Read the model definition and answer for the solid it produces. Units are mm, in the model's axes. A direction names the side the tool comes from. Give positions to 0.01 mm unless a question says otherwise; leave off trailing zeros. Loops run counter-clockwise (first coordinate to the right, second up) from the corner with the lowest first, then second, coordinate; pieces in that order, holes last. Notation, with made-up numbers: (48, 31.5) - (77, 31.5) arc R24 ccw to (77, 47.5) - close; hole circle Ø5 at (44.25, 70). An arc over 180 degrees is marked (long way). Put each result on its own line as item: value. Start each with the question number.
1. A cutting plane is placed at B-B, the plane x = 0. Determine the outline of the cut face in (y, z).
2. Given pin 1 Ø3 at (x, z) = (1.5, 74.5) entering from +Y; pin 2 Ø3 at (x, z) = (-1, 29.5) entering from -Y; pin 3 Ø6 at (y, z) = (-0.5, 71) entering from -X, each flat-ended and moving along its own axis, determine where each tip first touches the part or whether it passes through.
3. A cutting plane is placed at A-A, the plane y = -20. Determine the outline of the cut face in (x, z), plus the area to 3 significant figures.
4. For a pull along X with two mould halves and no side action, classify faces 1 (the flat face through (-3.901, 0, 49)), 2 (the flat face through (-8.2, -4, 49)), 3 (the flat face through (-4, 8.2, 49)), 4 (the flat face through (10, -10, 49)) as released by +X, released by -X, zero draft, split by the parting line, or undercut.
5. For faces 5 (the flat face through (0, -23.901, 49)), 6 (the flat face through (-9.11, -16.25, 49.3)), 7 (the flat face through (-7, -13.001, 51)), 8 (the flat face through (3.901, -20, 49)), determine the directions among +Z, -Z, +X, -X, +Y, -Y from which every point of the face is accessible in a straight line to the end or side of a thin tool.
6. Consider L1, parallel to Y at x = 0, z = 79.5; L2, parallel to Y at x = 6, z = 60; L3, parallel to Y at x = -5.25, z = 56. Determine where each line is inside the solid, lowest interval first. Write a range as from..to.
7. A cutting plane is placed at C-C, the plane z = 53. Count the separate pieces of the cut face and the enclosed holes in it, plus the area to 3 significant figures.
Autodesk Inventor part; units mm, degrees
ref_plane "Work Plane3" through (0, -20, 0) normal (0, 1, 0) x (-1, 0, 0)
ref_plane "YZ Plane" through (0, 0, 0) normal (1, 0, 0) x (0, 1, 0)
ref_plane "XY Plane" through (0, 0, 0) normal (0, 0, 1) x (1, 0, 0)
sketch "Sketch1" plane through (0, 0, 0) normal (0, 0, 1) x (1, 0, 0)
  line L0 (-3.9007, 3.9007) -> (3.9007, 3.9007)
  line L1 (3.9007, 3.9007) -> (3.9007, -3.9007)
  line L2 (3.9007, -3.9007) -> (-3.9007, -3.9007)
  line L3 (-3.9007, -3.9007) -> (-3.9007, 3.9007)
  line L4 (0, 3.9007) -> (0, -3.9007) construction
  line L5 (-3.9007, 0) -> (3.9007, 0) construction
  circle A0 centre (0, 0) radius 2.1
  line L6 (0, 0) -> (-16.1173, 16.1173) construction
  line L7 (0, 0) -> (22.7933, 0) construction
  line L8 (-2.84, 3.9007) -> (-5.4993, 6.56)
  line L9 (-5.4993, 6.56) -> (-5.4993, 8.2)
  line L10 (-5.4993, 8.2) -> (-2.84, 8.2)
  line L11 (-2.84, 8.2) -> (-4.64, 10)
  line L12 (-4.64, 10) -> (-10, 10)
  line L13 (-10, 10) -> (-10, 4.64)
  line L14 (-10, 4.64) -> (-8.2, 2.84)
  line L15 (-8.2, 2.84) -> (-8.2, 5.4993)
  line L16 (-8.2, 5.4993) -> (-6.56, 5.4993)
  line L17 (-6.56, 5.4993) -> (-3.9007, 2.84)
  line L18 (-3.9007, 2.84) -> (-11.3102, 2.84) construction
  line L19 (-2.84, 3.9007) -> (-3.9007, 3.9007)
  line L20 (-3.9007, 2.84) -> (-3.9007, 3.9007)
  line L21 (-3.9007, -2.84) -> (-6.56, -5.4993)
  line L22 (-6.56, -5.4993) -> (-8.2, -5.4993)
  line L23 (-8.2, -5.4993) -> (-8.2, -2.84)
  line L24 (-8.2, -2.84) -> (-10, -4.64)
  line L25 (-10, -4.64) -> (-10, -10)
  line L26 (-10, -10) -> (-4.64, -10)
  line L27 (-4.64, -10) -> (-2.84, -8.2)
  line L28 (-2.84, -8.2) -> (-5.4993, -8.2)
  line L29 (-5.4993, -8.2) -> (-5.4993, -6.56)
  line L30 (-5.4993, -6.56) -> (-2.84, -3.9007)
  line L31 (-3.9007, -2.84) -> (-3.9007, -3.9007)
  line L32 (-2.84, -3.9007) -> (-3.9007, -3.9007)
  line L33 (2.84, -3.9007) -> (5.4993, -6.56)
  line L34 (5.4993, -6.56) -> (5.4993, -8.2)
  line L35 (5.4993, -8.2) -> (2.84, -8.2)
  line L36 (2.84, -8.2) -> (4.64, -10)
  line L37 (4.64, -10) -> (10, -10)
  line L38 (10, -10) -> (10, -4.64)
  line L39 (10, -4.64) -> (8.2, -2.84)
  line L40 (8.2, -2.84) -> (8.2, -5.4993)
  line L41 (8.2, -5.4993) -> (6.56, -5.4993)
  line L42 (6.56, -5.4993) -> (3.9007, -2.84)
  line L43 (2.84, -3.9007) -> (3.9007, -3.9007)
  line L44 (3.9007, -2.84) -> (3.9007, -3.9007)
  line L45 (3.9007, 2.84) -> (6.56, 5.4993)
  line L46 (6.56, 5.4993) -> (8.2, 5.4993)
  line L47 (8.2, 5.4993) -> (8.2, 2.84)
  line L48 (8.2, 2.84) -> (10, 4.64)
  line L49 (10, 4.64) -> (10, 10)
  line L50 (10, 10) -> (4.64, 10)
  line L51 (4.64, 10) -> (2.84, 8.2)
  line L52 (2.84, 8.2) -> (5.4993, 8.2)
  line L53 (5.4993, 8.2) -> (5.4993, 6.56)
  line L54 (5.4993, 6.56) -> (2.84, 3.9007)
  line L55 (3.9007, 2.84) -> (3.9007, 3.9007)
  line L56 (2.84, 3.9007) -> (3.9007, 3.9007)
  dimension "d7" = 4.2
  dimension "d8" = 135
  dimension "d9" = 1.5
  dimension "d10" = 1.64
  dimension "d11" = 1.8
  dimension "d12" = 2.84
  dimension "d13" = 10
  dimension "d16" = 360
extrude "Extrusion1" add sketch "Sketch1" along normal blind 100
pattern_linear "Rectangular Pattern1" count 2 spacing 20 along (0, -1, 0) of "Extrusion1"
sketch "Sketch2" plane through (0, 0, 100) normal (0, 0, 1) x (1, 0, 0)
  line L0 (8.2, -2.84) -> (8.2, -5.4993)
  line L1 (8.2, -5.4993) -> (6.56, -5.4993)
  line L2 (-6.56, -5.4993) -> (-8.2, -5.4993)
  line L3 (-8.2, -5.4993) -> (-8.2, -2.84)
  line L4 (-8.2, -14.5007) -> (-6.56, -14.5007)
  line L5 (6.56, -14.5007) -> (8.2, -14.5007)
  line L6 (5.4993, -11.8) -> (5.4993, -13.44)
  line L7 (5.4993, -13.44) -> (2.84, -16.0993)
  line L8 (-2.84, -16.0993) -> (-5.4993, -13.44)
  line L9 (-5.4993, -8.2) -> (-5.4993, -6.56)
  line L10 (-5.4993, -6.56) -> (-2.84, -3.9007)
  line L11 (2.84, -3.9007) -> (5.4993, -6.56)
  line L12 (2.84, -8.2) -> (4.64, -10)
  line L13 (-8.2, -6.9993) -> (-5.9387, -6.9993)
  line L14 (-5.9387, -6.9993) -> (-4.1231, -5.1837)
  line L15 (-4.1231, -5.1837) -> (4.1231, -5.1837)
  line L16 (4.1231, -5.1837) -> (5.9387, -6.9993)
  line L17 (5.9387, -6.9993) -> (8.2, -6.9993)
  line L18 (8.2, -6.9993) -> (8.2, -13.0007)
  line L19 (8.2, -13.0007) -> (5.9387, -13.0007)
  line L20 (5.9387, -13.0007) -> (4.2461, -14.6932)
  line L21 (4.2461, -14.6932) -> (-4.2461, -14.6932)
  line L22 (-4.2461, -14.6932) -> (-5.9387, -13.0007)
  line L23 (-5.9387, -13.0007) -> (-8.2, -13.0007)
  line L24 (-8.2, -13.0007) -> (-8.2, -6.9993)
  dimension "d23" = 1.5
  dimension "d24" = 1.5
  dimension "d25" = 1.5
  dimension "d26" = 1.5
extrude "Extrusion2" cut sketch "Sketch2" against normal up to next
ref_plane "Work Plane3" through (0, -20, 0) normal (0, 1, 0) x (-1, 0, 0)
ref_plane "Work Plane2" through (0, 0, 0) normal (0, 1, 0) x (-1, 0, 0)
ref_plane "Work Plane1" through (0, -10, 0) normal (0, 1, 0) x (-1, 0, 0)
equation "\"d24\" = d23"
equation "\"d25\" = d23"
equation "\"d26\" = d23"
properties part number "20x40x597mm" material "Aluminum 6061"
Return value:
1. outline: (-23.9, 0) - (-22.1, 0) - (-22.1, 100) - (-23.9, 100) - close; (-17.9, 0) - (-16.1, 0) - (-16.1, 100) - (-17.9, 100) - close; (-3.9, 0) - (-2.1, 0) - (-2.1, 100) - (-3.9, 100) - close; (2.1, 0) - (3.9, 0) - (3.9, 100) - (2.1, 100) - close
2. pin 1: stops at y = 8.36
2. pin 2: stops at y = -23.9
2. pin 3: stops at x = -8.86
3. outline: (-3.9, 0) - (-2.1, 0) - (-2.1, 100) - (-3.9, 100) - close; (2.1, 0) - (3.9, 0) - (3.9, 100) - (2.1, 100) - close
3. area: 360 mm2
4. face 1: released by -X
4. face 2: undercut
4. face 3: undercut
4. face 4: released by +X
5. face 5: +Z, -Z, -Y
5. face 6: +Z, -Z, -X
5. face 7: +Z, -Z
5. face 8: +Z, -Z, +X
6. L1: y = -23.9..-22.1, -17.9..-16.1, -3.9..-2.1, 2.1..3.9
6. L2: y = -30..-24.94, -15.06..-13, -7..-4.94, 4.94..10
6. L3: y = -30..-28.2, -26.31..-24.19, -15.81..-13.69, -6.31..-4.19, 4.19..6.31, 8.2..10
7. separate pieces: 1
7. enclosed holes: 3
7. area: 297 mm2
